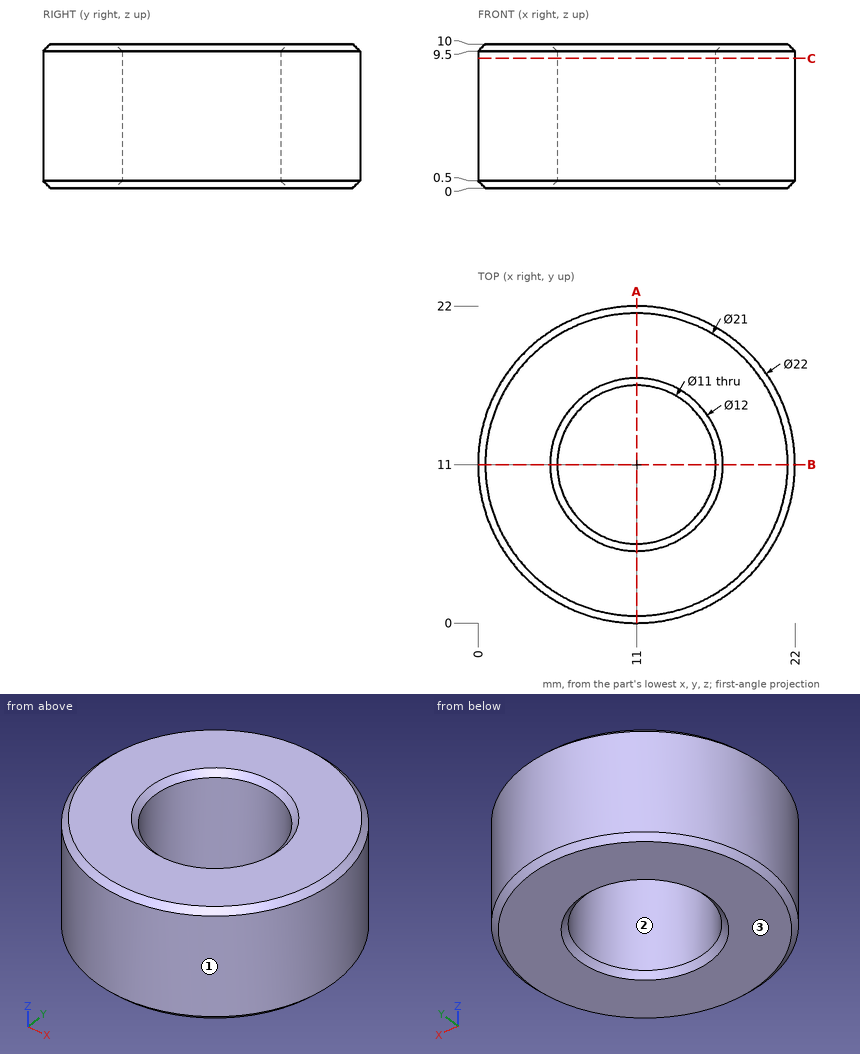
Job drawing, mm, ordinate dimensions from the low corner. One solid piece. Give positions to 0.01 mm unless a question says otherwise; leave off trailing zeros. Order: outer loops, then holes, each group sorted by start corner. A loop starts at its lowest first (then second) coordinate and runs counter-clockwise, first axis right, second up. Notation, with made-up numbers: M -26,70.25 L 30,70.25 A21 cw 30,95.25 Z; hole C 23.25,5 d11. An arc over 180 degrees is marked long. Return JSON: item names as keys, results as strings.
Q1. Wall check: probe 1 along Y at (x, z) = (11, 2.75); probe 2 along X at (y, z) = (15.25, 2.75); probe 3 along Y at (x, z) = (15.5, 3.5). Give the ranges that are in metal, low to high. Write a range as from..to.
Answer list:
{"probe 1": "y = 0..5.5, 16.5..22", "probe 2": "x = 0.85..7.51, 14.49..21.15", "probe 3": "y = 0.96..7.84, 14.16..21.04"}
Q2. Band-saw the part on C-C (z = 9). Give the cut face in (x, y), then the cut area to 3 significant figures.
Answer list:
{"outline": "C 11,11 d22; hole C 11,11 d11", "area": "285 mm^2"}
Q3. Two-plate mould, pull along Y, no slides. Class the marked faces 1, 2 and 3: pulls with the +Y half, pulls with the -Y half, needs draft (parallel to the pull), parting line crosses it, or undercut.
Answer list:
{"face 1": "parting line crosses it", "face 2": "undercut", "face 3": "needs draft"}
Q4. Flat gauge pins, fed straight in: pin 1 (4 mm diameter, centred on x = 8, z = 8, fed in from -Y); pin 2 (4 mm diameter, centred on x = 14.5, z = 2.5, fed in from -Y); pin 3 (1.5 mm diameter, centred on y = 7.5, z = 6, fed in from +X). Where does each tip first touch, or does it go through?
Answer list:
{"pin 1": "stops at y = 0.05", "pin 2": "stops at y = 0.1", "pin 3": "stops at x = 21.65"}
Q5. Band-saw the part on A-A (x = 11). Give the cut face in (y, z), then the cut area to 3 significant figures.
Answer list:
{"outline": "M 0,0.5 L 0.5,0 L 5,0 L 5.5,0.5 L 5.5,9.5 L 5,10 L 0.5,10 L 0,9.5 Z; M 16.5,0.5 L 17,0 L 21.5,0 L 22,0.5 L 22,9.5 L 21.5,10 L 17,10 L 16.5,9.5 Z", "area": "109 mm^2"}
